from build123d import *

# Parameters (mm, degrees)
SKETCH_1_R          = 2.35
EXTRUDE_1_DEPTH     = 18
SKETCH_3_R          = 3.5
EXTRUDE_2_DEPTH     = 3
CUT_EXTRUDE_2_DEPTH = 5


with BuildPart() as part:
    # 스케치1 → 보스-돌출1 (new body)
    with BuildSketch(Plane(origin=(0, 0, 0), x_dir=(1, 0, 0), z_dir=(0, 1, 0))):
        with Locations(Location((0, 0, 0), (0, 0, 270))):
            Circle(SKETCH_1_R)
    extrude(amount=EXTRUDE_1_DEPTH)

    # 스케치3 → 보스-돌출2 (add)
    with BuildSketch(Plane(origin=(0, 0, 0), x_dir=(-1, 0, 0), z_dir=(0, -1, 0))):
        with Locations(Location((0, 0, 0), (0, 0, 90))):
            Circle(SKETCH_3_R)
    extrude(amount=EXTRUDE_2_DEPTH)

    # 스케치6 → 컷-돌출2 (cut)
    with BuildSketch(Plane(origin=(0, 18, 0), x_dir=(1, 0, 0), z_dir=(0, 1, 0))):
        Polygon((1.99637355, 1.320619816), (-1.996753764, 1.320619816), (-2.00362645, 2.467115277), (1.99637355, 2.467115277), align=None)
        Polygon((1.99637355, -2.467115277), (1.99637355, -1.320619816), (-1.996753764, -1.320619816), (-2.00362645, -2.467115277), align=None)
    extrude(amount=-CUT_EXTRUDE_2_DEPTH, mode=Mode.SUBTRACT)


solid = part.part
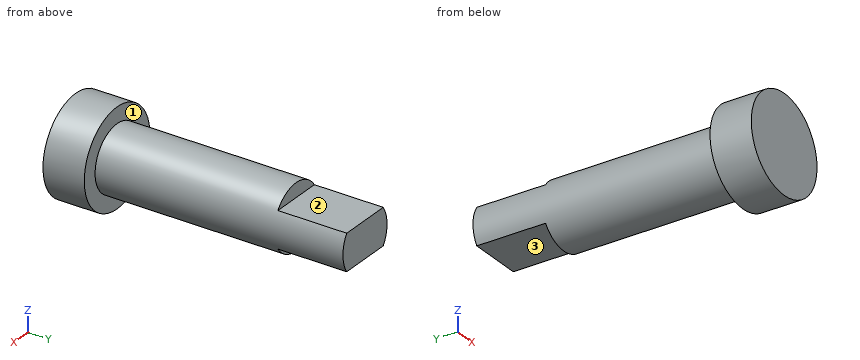
For this review, take the finished solid that the model builds, in its own axes (mm). Face numbers are marked on the shaded views. A direction names the side the tool comes from. Coordinates: 2 decimals unless noted, no trailing zeros. Loops run counter-clockwise (first coordinate to the right, second up) from the corner with the lowest first, then second, coordinate; pieces in that order, holes last. Notation, with made-up numbers: (52.5, 19.5) - (82.5, 19.5) arc R12 cw to (82.5, 26.5) - close; hole circle Ø9 at (-38, -7.5). An arc over 180 degrees is marked (long way). Use a Markdown table: item, result. Add a question column.
Item 1: We need section B-B (z = 0). Give the boundary of the cut face in (x, y), and give its area (3 significant figures).
Item 2: We need section D-D (x = 1). Give the boundary of the cut face in (y, z), and give its area (3 significant figures).
Item 3: Tool access review of the marked faces 1, 2 and 3: name each direction out of +Z, -Z, +X, -X, +Y, -Y from which nothing blocks a thin tool from reaching the whole face with its end or side.
Item 4: Insertion check: pin 1 Ø2 at (x, z) = (1, 1.5) entering from +Y; pin 2 Ø1.2 at (x, y) = (-0.5, 15) entering from -Z; pin 3 Ø3 at (x, y) = (0, 3.5) entering from -Z; pin 4 Ø1.9 at (x, y) = (0.5, 16) entering from +Z. Each pin has a flat end and moves straight along its axis. Give the tip position at first contact, or say it passes through.
Item 5: We need section C-C (y = -0.5). Give the boundary of the cut face in (x, z), and give its area (3 significant figures).
Item 6: We need section A-A (x = 0). Give the boundary of the cut face in (y, z), and give its area (3 significant figures).
Item 7: For line 1 (Y direction, x = 0, z = -1.5); line 2 (Y direction, x = -1.5, z = -2.25); line 3 (Z direction, x = 0, y = 11), list the stretches that pass through material, from the lowest coordinate up.
Results list:
| question | item | result |
|---|---|---|
| 1 | outline | (-3.5, -3) - (3.5, -3) - (3.5, 0) - (2.35, 0) - (2.35, 18) - (-2.35, 18) - (-2.35, 0) - (-3.5, 0) - close |
| 1 | area | 106 mm^2 |
| 2 | outline | (-3, -3.35) - (0, -3.35) - (0, -2.13) - (13, -2.13) - (13, -1.32) - (18, -1.32) - (18, 1.32) - (13, 1.32) - (13, 2.13) - (0, 2.13) - (0, 3.35) - (-3, 3.35) - close |
| 2 | area | 88.6 mm^2 |
| 3 | face 1 | +Y |
| 3 | face 2 | +Z, +X, -X, +Y |
| 3 | face 3 | -Z, +X, -X, +Y |
| 4 | pin 1 | stops at y = 18 |
| 4 | pin 2 | stops at z = -1.32 |
| 4 | pin 3 | stops at z = -2.35 |
| 4 | pin 4 | stops at z = 1.32 |
| 5 | outline | circle Ø7 at (0, 0) |
| 5 | area | 38.5 mm^2 |
| 6 | outline | (-3, -3.5) - (0, -3.5) - (0, -2.35) - (13, -2.35) - (13, -1.32) - (18, -1.32) - (18, 1.32) - (13, 1.32) - (13, 2.35) - (0, 2.35) - (0, 3.5) - (-3, 3.5) - close |
| 6 | area | 95.3 mm^2 |
| 7 | line 1 | y = -3 to 13 |
| 7 | line 2 | y = -3 to 0 |
| 7 | line 3 | z = -2.35 to 2.35 |
